The model under review builds one solid part; all positions refer to its coordinate system, in mm. A direction names the side the tool comes from. Coordinates: 2 decimals unless noted, no trailing zeros. Loops run counter-clockwise (first coordinate to the right, second up) from the corner with the lowest first, then second, coordinate; pieces in that order, holes last. Notation, with made-up numbers: M -13.5,-25.75 L 8.5,-25.75 A18 cw 8.5,-10.75 Z; hole C -4.5,48 d2. An arc over 180 degrees is marked long. Use CSV: the item, a comma, the result in double quotes. Start each with the question number.
1. Add section C-C, the plane y = -29. Write out the cut boundary in (x, z), then the cut area to 3 significant figures.
2. Draft analysis for pull direction Z (two halves, no side actions). For faces 3 (the flat face through (23, -63.5, -35)), 4 (the cylindrical face through (-8.361, -19.672, -37.653)), 5 (the flat face through (-1, 0, -74.892)), state which applies: +Z half, -Z half, draft (parallel to the pull), parting line (faces both ways), or undercut.
3. Add section A-A, the plane z = 0. Write out the cut boundary in (x, y).
4. For L1, parallel to Z at x = 0, y = -5; L2, parallel to Z at x = 0, y = -31.5; L3, parallel to X at y = 7.5, z = -34, list the stretches that pass through material, from the lowest coordinate up.
5. Add section B-B, the plane x = 0. Write out the cut boundary in (y, z), then the cut area to 3 significant figures.
6. Tool access review of faces 1 (the flat face through (-18, 25.4, 34.3)), 2 (the flat face through (-52, -25.4, 18)): name each direction out of +Z, -Z, +X, -X, +Y, -Y from which nothing blocks a thin tool from reaching the whole face with its end or side.
7. Add section D-D, the plane x = 59.5. Write out the cut boundary in (y, z).
from build123d import *

# Parameters (mm, degrees)
F0_W          = 152.688384
F0_H          = 149.784088
F1_DEPTH      = 25.4
F1_DEPTH_BACK = 25.4
F2_R          = 53.622423
F3_DEPTH      = 38.1
F4_R          = 38.570036
F5_DEPTH      = 127


with BuildPart() as f1:
    # F0 (on Front) → F1 (new body, two sides)
    with BuildSketch(Plane.XZ) as f1_sk:
        Rectangle(F0_W, F0_H)
    extrude(amount=F1_DEPTH)
    extrude(f1_sk.sketch, amount=-F1_DEPTH_BACK)

    # F2 (on face) → F3 (join)
    with BuildSketch(Plane.XZ.offset(25.4)):
        Circle(F2_R)
    extrude(amount=F3_DEPTH)

    # F4 (on face) → F5 (cut)
    with BuildSketch(Plane.XZ.offset(63.5)):
        Circle(F4_R)
    extrude(amount=-F5_DEPTH, mode=Mode.SUBTRACT)


solid = f1.part
Computed:
1,outline,"C 0,0 d107.24; hole C 0,0 d77.14"
1,area,"4,360 mm^2"
2,face 3,"draft"
2,face 4,"undercut"
2,face 5,"-Z half"
3,outline,"M -76.34,-25.4 L -53.62,-25.4 L -53.62,-63.5 L -38.57,-63.5 L -38.57,25.4 L -76.34,25.4 Z; M 38.57,-63.5 L 53.62,-63.5 L 53.62,-25.4 L 76.34,-25.4 L 76.34,25.4 L 38.57,25.4 Z"
4,L1,"z = -74.89 to -38.57, 38.57 to 74.89"
4,L2,"z = -53.62 to -38.57, 38.57 to 53.62"
4,L3,"x = -76.34 to -18.21, 18.21 to 76.34"
5,outline,"M -63.5,-53.62 L -25.4,-53.62 L -25.4,-74.89 L 25.4,-74.89 L 25.4,-38.57 L -63.5,-38.57 Z; M -63.5,38.57 L 25.4,38.57 L 25.4,74.89 L -25.4,74.89 L -25.4,53.62 L -63.5,53.62 Z"
5,area,"4,840 mm^2"
6,face 1,"+Z, -Z, +X, -X, +Y"
6,face 2,"-Y"
7,outline,"M -25.4,-74.89 L 25.4,-74.89 L 25.4,74.89 L -25.4,74.89 Z"
